CAD build for the part. Positions are in the model's coordinates, mm. A direction names the side the tool comes from. Coordinates: 2 decimals unless noted, no trailing zeros. Order: outer loops, then holes, each group sorted by start corner. A loop starts at its lowest first (then second) coordinate and runs counter-clockwise, first axis right, second up. Notation, with made-up numbers: (51, 75) - (56, 75) arc R12 ccw to (56, 97) - close; hole circle Ø9 at (69.25, 88). An arc over 180 degrees is marked (long way). Use one line per item in the form item = value.
```python
from build123d import *

# Parameters (mm, degrees)
F0_R      = 34.95
F0_R_2    = 24.925
F0_W      = 11.2
F0_H      = 11.2
F0_R_3    = 1.6
F0_R_4    = 3
F1_DEPTH  = 10
F2_R      = 0.5
F3_DEPTH  = 4.5
F4_DEPTH  = 4.75
F5_R      = 4
F5_R_2    = 1.6
F6_DEPTH  = 34.25
F7_DEPTH  = 3
F8_W      = 11.2
F8_H      = 11.2
F8_R      = 3
F8_R_2    = 1.6
F9_DEPTH  = 5.5
F10_DEPTH = 35.94117
F11_DEPTH = 8


# Not quite as in the source:
# - a feature names something its author has since deleted; it is built from what else it names


with BuildPart() as f1:
    # F0 (on Top) → F1 (new body)
    with BuildSketch(Plane.XY):
        with Locations((30.3336817496, -8.5733028001)):
            Circle(F0_R)
        with Locations((30.3336817496, -8.5733028001)):
            Circle(F0_R_2, mode=Mode.SUBTRACT)
        with Locations((30.3336817496, -8.5733028001)):
            Circle(F0_R_2)
        Polygon((18.1502625033, -17.7733028001), (19.766843257, -20.5733028001), (18.1502625033, -23.3733028001), (14.9171009958, -23.3733028001), (13.3005202421, -20.5733028001), (14.9171009958, -17.7733028001), align=None, mode=Mode.SUBTRACT)
        Polygon((45.7502625033, -17.7733028001), (47.366843257, -20.5733028001), (45.7502625033, -23.3733028001), (42.5171009958, -23.3733028001), (40.9005202421, -20.5733028001), (42.5171009958, -17.7733028001), align=None, mode=Mode.SUBTRACT)
        Polygon((42.5171009958, -11.3733028001), (40.9005202421, -8.5733028001), (42.5171009958, -5.7733028001), (45.7502625033, -5.7733028001), (47.366843257, -8.5733028001), (45.7502625033, -11.3733028001), align=None, mode=Mode.SUBTRACT)
        Polygon((14.9171009958, -11.3733028001), (13.3005202421, -8.5733028001), (14.9171009958, -5.7733028001), (18.1502625033, -5.7733028001), (19.766843257, -8.5733028001), (18.1502625033, -11.3733028001), align=None, mode=Mode.SUBTRACT)
        with Locations((30.3336817496, -8.5733028001)):
            Rectangle(F0_W, F0_H, mode=Mode.SUBTRACT)
        Polygon((42.5171009958, -5.7733028001), (40.9005202421, -8.5733028001), (42.5171009958, -11.3733028001), (45.7502625033, -11.3733028001), (47.366843257, -8.5733028001), (45.7502625033, -5.7733028001), align=None)
        with Locations((44.1336817496, -8.5733028001)):
            Circle(F0_R_3, mode=Mode.SUBTRACT)
        Polygon((45.7502625033, -23.3733028001), (47.366843257, -20.5733028001), (45.7502625033, -17.7733028001), (42.5171009958, -17.7733028001), (40.9005202421, -20.5733028001), (42.5171009958, -23.3733028001), align=None)
        with Locations((44.1336817496, -20.5733028001)):
            Circle(F0_R_3, mode=Mode.SUBTRACT)
        Polygon((18.1502625033, -23.3733028001), (19.766843257, -20.5733028001), (18.1502625033, -17.7733028001), (14.9171009958, -17.7733028001), (13.3005202421, -20.5733028001), (14.9171009958, -23.3733028001), align=None)
        with Locations((16.5336817496, -20.5733028001)):
            Circle(F0_R_3, mode=Mode.SUBTRACT)
        Polygon((14.9171009958, -5.7733028001), (13.3005202421, -8.5733028001), (14.9171009958, -11.3733028001), (18.1502625033, -11.3733028001), (19.766843257, -8.5733028001), (18.1502625033, -5.7733028001), align=None)
        with Locations((16.5336817496, -8.5733028001)):
            Circle(F0_R_3, mode=Mode.SUBTRACT)
        with Locations((30.3336817496, -8.5733028001)):
            Rectangle(F0_W, F0_H)
        with Locations((30.3336817496, -8.5733028001)):
            Circle(F0_R_4, mode=Mode.SUBTRACT)
        with Locations((30.3336817496, -8.5733028001)):
            Circle(F0_R_4)
        with Locations((30.3336817496, -8.5733028001)):
            Circle(F0_R_3, mode=Mode.SUBTRACT)
    extrude(amount=F1_DEPTH)

    # F2
    f2_edges = [f1.edges().sort_by_distance(p)[0] for p in [
        (-4.616318, -8.573303, 10),
    ]]
    fillet(f2_edges, radius=F2_R)

    # F0 (on Top) → F3 (join)
    with BuildSketch(Plane.XY):
        with Locations((30.3336817496, -8.5733028001)):
            Rectangle(F0_W, F0_H)
        with Locations((30.3336817496, -8.5733028001)):
            Circle(F0_R_4, mode=Mode.SUBTRACT)
        Polygon((18.1502625033, -23.3733028001), (19.766843257, -20.5733028001), (18.1502625033, -17.7733028001), (14.9171009958, -17.7733028001), (13.3005202421, -20.5733028001), (14.9171009958, -23.3733028001), align=None)
        with Locations((16.5336817496, -20.5733028001)):
            Circle(F0_R_3, mode=Mode.SUBTRACT)
        Polygon((45.7502625033, -23.3733028001), (47.366843257, -20.5733028001), (45.7502625033, -17.7733028001), (42.5171009958, -17.7733028001), (40.9005202421, -20.5733028001), (42.5171009958, -23.3733028001), align=None)
        with Locations((44.1336817496, -20.5733028001)):
            Circle(F0_R_3, mode=Mode.SUBTRACT)
    extrude(amount=F3_DEPTH)

    # F0 (on Top) → F4 (cut)
    with BuildSketch(Plane.XY):
        with Locations((30.3336817496, -8.5733028001)):
            Circle(F0_R)
        with Locations((30.3336817496, -8.5733028001)):
            Circle(F0_R_2, mode=Mode.SUBTRACT)
    extrude(amount=F4_DEPTH, mode=Mode.SUBTRACT)

    # F5 (on face) + F0 (on Top) → F6 (join)
    with BuildSketch(Plane(origin=(0, 0, 0), x_dir=(1, 0, 0), z_dir=(0, 0, -1))):
        with Locations((30.3336817496, 8.5733028001)):
            Circle(F5_R)
        with Locations((30.3336817496, 8.5733028001)):
            Circle(F5_R_2, mode=Mode.SUBTRACT)
    with BuildSketch(Plane.XY):
        with Locations((30.3336817496, -8.5733028001)):
            Circle(F0_R_4)
        with Locations((30.3336817496, -8.5733028001)):
            Circle(F0_R_3, mode=Mode.SUBTRACT)
    extrude(amount=F6_DEPTH, dir=(0, 0, -1))

    # F0 (on Top) → F7 (cut)
    with BuildSketch(Plane.XY):
        Polygon((45.7502625033, -23.3733028001), (47.366843257, -20.5733028001), (45.7502625033, -17.7733028001), (42.5171009958, -17.7733028001), (40.9005202421, -20.5733028001), (42.5171009958, -23.3733028001), align=None)
        with Locations((44.1336817496, -20.5733028001)):
            Circle(F0_R_3, mode=Mode.SUBTRACT)
        Polygon((42.5171009958, -5.7733028001), (40.9005202421, -8.5733028001), (42.5171009958, -11.3733028001), (45.7502625033, -11.3733028001), (47.366843257, -8.5733028001), (45.7502625033, -5.7733028001), align=None)
        with Locations((44.1336817496, -8.5733028001)):
            Circle(F0_R_3, mode=Mode.SUBTRACT)
        Polygon((14.9171009958, -5.7733028001), (13.3005202421, -8.5733028001), (14.9171009958, -11.3733028001), (18.1502625033, -11.3733028001), (19.766843257, -8.5733028001), (18.1502625033, -5.7733028001), align=None)
        with Locations((16.5336817496, -8.5733028001)):
            Circle(F0_R_3, mode=Mode.SUBTRACT)
        Polygon((18.1502625033, -23.3733028001), (19.766843257, -20.5733028001), (18.1502625033, -17.7733028001), (14.9171009958, -17.7733028001), (13.3005202421, -20.5733028001), (14.9171009958, -23.3733028001), align=None)
        with Locations((16.5336817496, -20.5733028001)):
            Circle(F0_R_3, mode=Mode.SUBTRACT)
    extrude(amount=F7_DEPTH, mode=Mode.SUBTRACT)

    # F8 (on face) → F9 (cut)
    with BuildSketch(Plane.XY.offset(10)):
        with Locations((30.3336817496, -8.5733028001)):
            Rectangle(F8_W, F8_H)
        with Locations((30.3336817496, -8.5733028001)):
            Circle(F8_R, mode=Mode.SUBTRACT)
        with Locations((30.3336817496, -8.5733028001)):
            Circle(F8_R)
        with Locations((30.3336817496, -8.5733028001)):
            Circle(F8_R_2, mode=Mode.SUBTRACT)
    extrude(amount=-F9_DEPTH, mode=Mode.SUBTRACT)

    # F0 (on Top) → F10 (cut)
    with BuildSketch(Plane.XY):
        with Locations((30.3336817496, -8.5733028001)):
            Circle(F0_R_3)
    extrude(amount=-F10_DEPTH, mode=Mode.SUBTRACT)

    # F8 (on face) → F11 (cut)
    with BuildSketch(Plane.XY.offset(10)):
        with Locations((30.3336817496, -8.5733028001)):
            Circle(F8_R)
        with Locations((30.3336817496, -8.5733028001)):
            Circle(F8_R_2, mode=Mode.SUBTRACT)
    extrude(amount=-F11_DEPTH, mode=Mode.SUBTRACT)


solid = f1.part
```
Item 1: Drill centre lines: line 1 (Z direction, x = 24, y = -12.5); line 2 (Z direction, x = 7.5, y = 9); line 3 (Y direction, x = 30, z = -26). Where is each one in solid material? Low to high. Write a range as [from, to].
Derived:
line_1 = [0, 10]
line_2 = [4.75, 10]
line_3 = [-12.56, -10.14], [-7.01, -4.59]
Item 2: 3-axis set-ups, long thin cutter, end or side, ignore diameter. For faces 1 (the face through (46.57, -19.19, 1.48)), 2 (the face through (32, -10, 2)), 3 (the face through (14.935, -8.503, 6.451)): which of +Z, -Z, +X, -X, +Y, -Y reach the whole face in a straight line?
Derived:
face_1 = -Z
face_2 = +Z
face_3 = +Z, -Z
Item 3: Drop flat-ended pins along their axis: pin 1 (2.5 mm diameter, centred on x = 44.5, z = 1, fed in from -Y); pin 2 (6 mm diameter, centred on y = -12, z = -24.5, fed in from +X); pin 3 (4.5 mm diameter, centred on x = 31, z = 8, fed in from -Y). Give the stop position or say it passes through.
Derived:
pin_1 = -29.89
pin_2 = 34.31
pin_3 = -43.52
Item 4: Two-plate mould, pull along Y, no slides. Class faces 4 (the face through (15.354, -19.492, 6.451)), 5 (the face through (42.954, -19.492, 6.451)), 6 (the face through (30, -16, 10)), 7 (the face through (34.15, -9.77, -16.89)): +Y half, -Y half, draft (parallel to the pull), parting line (faces both ways), or undercut.
Derived:
face_4 = undercut
face_5 = undercut
face_6 = draft
face_7 = parting line
Item 5: Cut at A-A, the plane z = -26. Write the cut outline in (x, y), plus the area to 3 significant figures.
Derived:
outline = circle Ø8 at (30.33, -8.57); hole circle Ø3.2 at (30.33, -8.57)
area = 42.2 mm²
